```python
from build123d import *

# Parameters (mm, degrees)
SKETCH1_W                = 15
SKETCH1_H                = 22
BOSS_EXTRUDE1_DEPTH      = 10
SKETCH2_W                = 12
SKETCH2_H                = 6
CUT_EXTRUDE1_DEPTH       = 50.771980069
SKETCH3_W                = 12
SKETCH3_H                = 6
CUT_EXTRUDE2_DEPTH       = 50.771980069
F_4_0_4_DIAMETER_HOLE1_D = 4


with BuildPart() as part:
    # Sketch1 → Boss-Extrude1 (new body)
    with BuildSketch(Plane(origin=(0, 0, 15), x_dir=(-1, 0, 0), z_dir=(0, 0, -1))):
        with Locations((40, 0)):
            Rectangle(SKETCH1_W, SKETCH1_H)
    extrude(amount=-BOSS_EXTRUDE1_DEPTH)

    # Sketch2 → Cut-Extrude1 (cut, through all)
    with BuildSketch(Plane.XY.offset(25)):
        with Locations((-41.5, 8)):
            Rectangle(SKETCH2_W, SKETCH2_H)
    extrude(amount=-CUT_EXTRUDE1_DEPTH, mode=Mode.SUBTRACT)

    # Sketch3 → Cut-Extrude2 (cut, through all)
    with BuildSketch(Plane.XY.offset(25)):
        with Locations((-41.5, -8)):
            Rectangle(SKETCH3_W, SKETCH3_H)
    extrude(amount=-CUT_EXTRUDE2_DEPTH, mode=Mode.SUBTRACT)

    # Sketch4 → Cut-Revolve1 (revolve, cut)
    with BuildSketch(Plane.XY.offset(20), mode=Mode.PRIVATE) as cut_revolve1_sk:
        Polygon((-35.5, 8.7835), (-35.5, 8), (-32.5, 8), (-32.5, 8.7835), (-34.5, 8.7835), align=None)
    revolve(cut_revolve1_sk.sketch.rotate(Axis((-35.5, 8, 20), (1, 0, 0)), 270), axis=Axis((-35.5, 8, 20), (1, 0, 0)), mode=Mode.SUBTRACT)

    # Sketch5 → Cut-Revolve2 (revolve, cut)
    with BuildSketch(Plane.XY.offset(20), mode=Mode.PRIVATE) as cut_revolve2_sk:
        Polygon((-35.5, -7.2165), (-35.5, -8), (-32.5, -8), (-32.5, -7.2165), (-34.5, -7.2165), align=None)
    revolve(cut_revolve2_sk.sketch.rotate(Axis((-35.5, -8, 20), (1, 0, 0)), 270), axis=Axis((-35.5, -8, 20), (1, 0, 0)), mode=Mode.SUBTRACT)

    # Ø4.0 (4) Diameter Hole1 (through all)
    with Locations(Plane(origin=(0, 0, 15), x_dir=(-1, 0, 0), z_dir=(0, 0, -1))):
        with Locations((38.7, 0)):
            Hole(F_4_0_4_DIAMETER_HOLE1_D / 2)


solid = part.part
```
Input: part model. Units: mm. Frame: model coordinates. A direction names the side the tool comes from. Give positions to 0.01 mm unless a question says otherwise; leave off trailing zeros. Order: outer loops, then holes, each group sorted by start corner. A loop starts at its lowest first (then second) coordinate and runs counter-clockwise, first axis right, second up. Notation, with made-up numbers: (38.25, 19) -> (46.25, 19) arc R22 ccw to (46.25, 44) -> close; hole circle Ø5 at (26.5, 81). An arc over 180 degrees is marked (long way). Write each question's results on one line, items separated by ' | '. Start each with the question number.
Item 1: Cut plane D-D on z = 22.5. Return the cut outline in (x, y).
Item 2: Cut plane C-C on x = -38.7. Return the cut outline in (y, z), then the cut area to 3 significant figures.
Item 3: Set-up query: faces 4 (the flat face through (-35.5, -8, 19)), 5 (the flat face through (-32.5, 0, 20)), 6 (the flat face through (-35.5, 8, 19)). Return all of +Z, -Z, +X, -X, +Y, -Y with unobstructed straight access to the full face (end or side cutting, diameter ignored); none if empty.
Item 4: Line query: line 1 (Y direction, x = -33.95, z = 20); line 2 (X direction, y = 9, z = 24); line 3 (Y direction, x = -38.7, z = 18). Output: solid intervals per line, ascending.
Item 5: Cut plane B-B on y = 8. Return the cut outline in (x, z).
Item 6: Mould query, pull axis Z, two halves, no side actions, for faces 1 (the flat face through (-42, 5, 20)), 2 (the flat face through (-38.2, -2.3, 25)), 3 (the cylindrical face through (-34.02, 7.52, 20.62)). Classes: pulls with the +Z half, pulls with the -Z half, needs draft (parallel to the pull), parting line crosses it, or undercut.
Item 7: Contact query for flat-ended pins moving along their axis: P1, Ø1.4, axis at y = -8, z = 20, coming from the -X side; P2, Ø3, axis at x = -40.5, z = 20, coming from the +Y side; P3, Ø6, axis at y = -8.5, z = 22, coming from the -X side. Output: stop coordinate, or through.
Item 8: Cut plane A-A on z = 20. Return the cut outline in (x, y).
Established:
1) outline: (-47.5, -5) -> (-35.5, -5) -> (-35.5, -11) -> (-32.5, -11) -> (-32.5, 11) -> (-35.5, 11) -> (-35.5, 5) -> (-47.5, 5) -> close; hole circle Ø4 at (-38.7, 0)
2) outline: (-5, 15) -> (-2, 15) -> (-2, 25) -> (-5, 25) -> close; (2, 15) -> (5, 15) -> (5, 25) -> (2, 25) -> close | area: 60.0 mm^2
3) face 4: +Z, -Z, -X, -Y | face 5: +Z, -Z, +X, +Y, -Y | face 6: +Z, -Z, -X, +Y
4) line 1: -11 to -8.78, -7.22 to 7.22, 8.78 to 11 | line 2: -35.5 to -32.5 | line 3: -5 to -2, 2 to 5
5) outline: (-35.5, 15) -> (-32.5, 15) -> (-32.5, 19.22) -> (-35.5, 19.22) -> close; (-35.5, 20.78) -> (-32.5, 20.78) -> (-32.5, 25) -> (-35.5, 25) -> close
6) face 1: needs draft | face 2: pulls with the +Z half | face 3: undercut
7) P1: through | P2: y = 5 | P3: x = -35.5
8) outline: (-47.5, -5) -> (-35.5, -5) -> (-35.5, -7.22) -> (-32.5, -7.22) -> (-32.5, 7.22) -> (-35.5, 7.22) -> (-35.5, 5) -> (-47.5, 5) -> close; (-35.5, -11) -> (-32.5, -11) -> (-32.5, -8.78) -> (-35.5, -8.78) -> close; (-35.5, 8.78) -> (-32.5, 8.78) -> (-32.5, 11) -> (-35.5, 11) -> close; hole circle Ø4 at (-38.7, 0)
